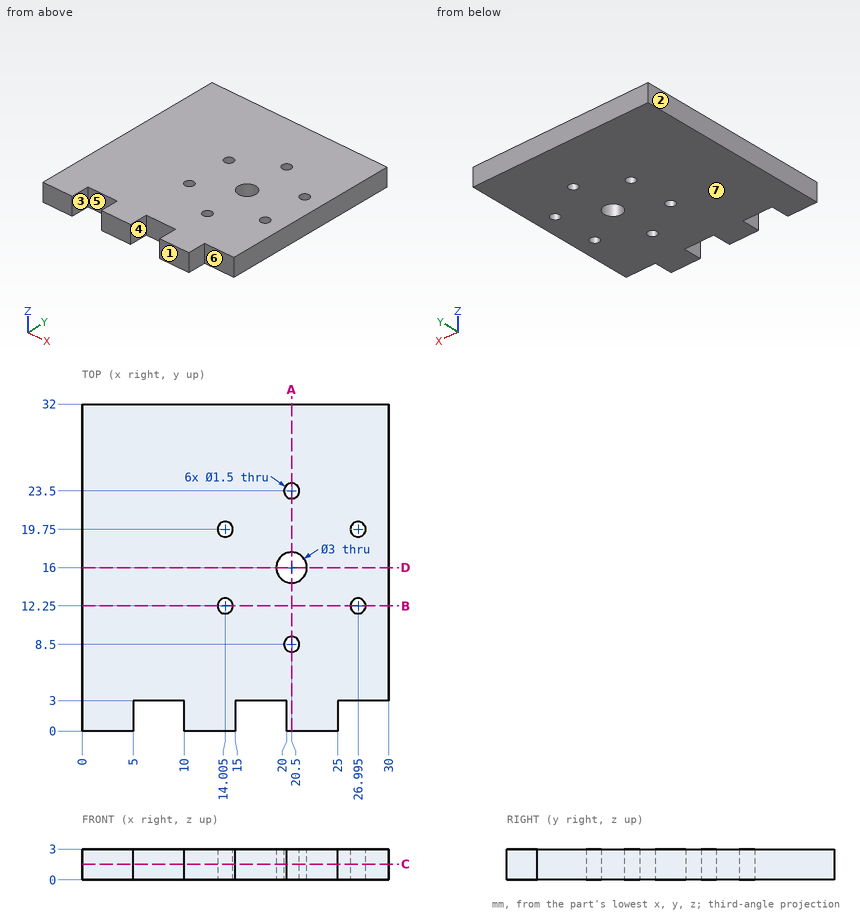
Design review of the part shown in the three views and the two pictorial views. Dimensions are in mm from the part's minimum x, y and z. A direction names the side the tool comes from. Coordinates: 2 decimals unless noted, no trailing zeros. Write each loop counter-clockwise with the first axis right and the second up, starting at its lowest first coordinate (ties: lowest second). Pieces come first, ordered by that corner, then holes.
(1) The part is to be moulded in two halves that separate along X. For the marked faces 1, 2, 3 and 4, say which applies: +X half, -X half, draft (parallel to the pull), parting line (faces both ways), or undercut.
(2) For pin 1 Ø1.5 at (y, z) = (1.5, 1) entering from +X; pin 2 Ø0.9 at (x, z) = (28, 1) entering from -Y, all flat-tipped, find the tip position at first contact; note any pin that passes through.
(3) Add section A-A on x = 20.5. Give the boundary of the cut face in (y, z), then the cut area to 3 significant figures.
(4) Add section B-B on y = 12.25. Give the boundary of the cut face in (x, z) (1 decimal).
(5) Add section C-C on z = 1.55. Count the separate pieces of the cut face and the enclosed holes in it, then the cut area to 3 significant figures.
(6) Tool access review of the marked faces 5, 6 and 7: name each direction out of +Z, -Z, +X, -X, +Y, -Y from which nothing blocks a thin tool from reaching the whole face with its end or side.
(7) Add section D-D on y = 16. Give the boundary of the cut face in (x, z).
(8) Wall thickness on probe 1 along Y at (x, z) = (14, 1.05); probe 2 along Y at (x, z) = (20.5, 2.2); probe 3 along Y at (x, z) = (27.5, 2.15) (1 decimal): over which ranges is each line inside the solid? List them lowest first.
Answer sheet:
1. face 1: draft
1. face 2: -X half
1. face 3: undercut
1. face 4: undercut
2. pin 1: stops at x = 25
2. pin 2: stops at y = 3
3. outline: (0, 0) - (7.75, 0) - (7.75, 3) - (0, 3) - close; (9.25, 0) - (14.5, 0) - (14.5, 3) - (9.25, 3) - close; (17.5, 0) - (22.75, 0) - (22.75, 3) - (17.5, 3) - close; (24.25, 0) - (32, 0) - (32, 3) - (24.25, 3) - close
3. area: 78.0 mm2
4. outline: (0, 0) - (13.3, 0) - (13.3, 3) - (0, 3) - close; (14.8, 0) - (26.2, 0) - (26.2, 3) - (14.8, 3) - close; (27.7, 0) - (30, 0) - (30, 3) - (27.7, 3) - close
5. separate pieces: 1
5. enclosed holes: 7
5. area: 897 mm2
6. face 5: +Z, -Z, -Y
6. face 6: +Z, -Z, +X, -Y
6. face 7: -Z, +X, -X, +Y, -Y
7. outline: (0, 0) - (19, 0) - (19, 3) - (0, 3) - close; (22, 0) - (30, 0) - (30, 3) - (22, 3) - close
8. probe 1: y = 0 to 11.5, 13 to 19, 20.5 to 32
8. probe 2: y = 0 to 7.75, 9.25 to 14.5, 17.5 to 22.75, 24.25 to 32
8. probe 3: y = 3 to 11.7, 12.8 to 19.2, 20.3 to 32
